```python
from build123d import *

# Parameters (mm, degrees)
SKETCH1_W           = 34.5
SKETCH1_H           = 60
BOSS_EXTRUDE1_DEPTH = 1
SKETCH2_W           = 38.5
SKETCH2_H           = 64
SKETCH2_W_2         = 34.5
SKETCH2_H_2         = 60
BOSS_EXTRUDE2_DEPTH = 17
SKETCH3_W           = 6
SKETCH3_H           = 3.2
CUT_EXTRUDE1_DEPTH  = 17
BOSS_EXTRUDE3_DEPTH = 2
SKETCH5_W           = 38.5
SKETCH5_H           = 64
SKETCH5_W_2         = 34.5
SKETCH5_H_2         = 60
BOSS_EXTRUDE4_DEPTH = 2
CHAMFER1_SIZE       = 2


with BuildPart() as part:
    # Sketch1 → Boss-Extrude1 (new body)
    with BuildSketch(Plane(origin=(0, 0, 0), x_dir=(1, 0, 0), z_dir=(0, 1, 0))):
        with Locations((17.25, 30)):
            Rectangle(SKETCH1_W, SKETCH1_H)
    extrude(amount=BOSS_EXTRUDE1_DEPTH)

    # Sketch2 → Boss-Extrude2 (add)
    with BuildSketch(Plane.XZ):
        with Locations((17.25, -30)):
            Rectangle(SKETCH2_W, SKETCH2_H)
        with Locations((17.25, -30)):
            Rectangle(SKETCH2_W_2, SKETCH2_H_2, mode=Mode.SUBTRACT)
    extrude(amount=-BOSS_EXTRUDE2_DEPTH)

    # Sketch3 → Cut-Extrude1 (cut)
    with BuildSketch(Plane(origin=(0, 0, 0), x_dir=(0, 0, -1), z_dir=(1, 0, 0))):
        with Locations((14.404129658, 2.6)):
            Rectangle(SKETCH3_W, SKETCH3_H)
    extrude(amount=-CUT_EXTRUDE1_DEPTH, mode=Mode.SUBTRACT)

    # Sketch4 → Boss-Extrude3 (add)
    with BuildSketch(Plane(origin=(0, 1, 0), x_dir=(1, 0, 0), z_dir=(0, 1, 0))):
        Polygon((0, 60), (34.5, 60), (34.5, 0), (0, 0), (0, 11.404129658), (20, 11.404129658), (20, 17.404129658), (0, 17.404129658), align=None)
    extrude(amount=BOSS_EXTRUDE3_DEPTH)

    # Sketch5 → Boss-Extrude4 (add)
    with BuildSketch(Plane(origin=(0, 17, 0), x_dir=(1, 0, 0), z_dir=(0, 1, 0))):
        with Locations((17.25, 30)):
            Rectangle(SKETCH5_W, SKETCH5_H)
        with Locations((17.25, 30)):
            Rectangle(SKETCH5_W_2, SKETCH5_H_2, mode=Mode.SUBTRACT)
    extrude(amount=BOSS_EXTRUDE4_DEPTH)

    # Chamfer1
    chamfer1_edges = [part.edges().sort_by_distance(p)[0] for p in [
        (20, 3, -14.404129658),
    ]]
    chamfer(chamfer1_edges, length=CHAMFER1_SIZE - 0.0001)  # a hair under: the kernel refuses the full size


solid = part.part
```
Check sheet for the modelled part. Datum: model origin and axes. Units: mm. A direction names the side the tool comes from. Coordinates: 2 decimals unless noted, no trailing zeros. Order: outer loops, then holes, each group sorted by start corner. A loop starts at its lowest first (then second) coordinate and runs counter-clockwise, first axis right, second up. Notation, with made-up numbers: M 44,73 L 50,73 A22 ccw 50,81 Z; hole C 89,7.25 d3. An arc over 180 degrees is marked long. One line per question, with ' | ' between items. Start each with the question number.
Item 1: Sectioned sample at C-C on x = 23.5. Record the cut outline in (y, z).
Item 2: Access from +Z, -Z, +X, -X, +Y, -Y to the whole of each face (thin tool, end or side, straight path). Record for faces 1 (the flat face through (17, 9, 2)), 2 (the flat face through (17, 11, -60)), 3 (the flat face through (-1, 4.2, -14)).
Item 3: Sectioned sample at B-B on y = 6.75. Record the cut outline in (x, z), and give its area (3 significant figures).
Item 4: Material ranges on line 1 (Z direction, x = 23, y = 8.25); line 2 (Z direction, x = 18, y = 2); line 3 (X direction, y = 14.5, z = -28.5), recorded low to high.
Item 5: Mould release check, pull along X, two halves, no side actions. Record for faces 4 (the flat face through (10, 2, -17.404)), 5 (the flat face through (21, 2, -14)), 6 (the flat face through (17, 3, -30)): pulls with the +X half, pulls with the -X half, needs draft (parallel to the pull), parting line crosses it, or undercut.
Item 6: Gauge pin test, flat ends, axial feed: P1, Ø3, axis at x = 13, z = -13, coming from the +Y side; P2, Ø8, axis at x = 11.5, z = -27, coming from the +Y side. Record the tip position at first contact, or that the pin passes through.
Item 7: Sectioned sample at D-D on z = -25.5. Record the cut outline in (x, y).
Answer below:
1) outline: M 0,-62 L 19,-62 L 19,-60 L 3,-60 L 3,0 L 19,0 L 19,2 L 0,2 Z
2) face 1: +Z, +X, -X, +Y, -Y | face 2: +Y | face 3: -X
3) outline: M -2,-62 L 36.5,-62 L 36.5,2 L -2,2 Z; hole M 0,-60 L 34.5,-60 L 34.5,0 L 0,0 Z | area: 394 mm^2
4) line 1: z = -62 to -60, 0 to 2 | line 2: z = -62 to -17.4, -11.4 to 2 | line 3: x = -2 to 0, 34.5 to 36.5
5) face 4: needs draft | face 5: pulls with the -X half | face 6: undercut
6) P1: stops at y = 1 | P2: stops at y = 3
7) outline: M -2,0 L 36.5,0 L 36.5,19 L 34.5,19 L 34.5,3 L 0,3 L 0,19 L -2,19 Z
